Geometry: final body of the model. Coordinates: model frame, mm. A direction names the side the tool comes from. Coordinates: 2 decimals unless noted, no trailing zeros. Order: outer loops, then holes, each group sorted by start corner. A loop starts at its lowest first (then second) coordinate and runs counter-clockwise, first axis right, second up. Notation, with made-up numbers: M 21.25,30.25 L 33.25,30.25 A23 ccw 33.25,38.25 Z; hole C 15.25,58.5 d3. An arc over 180 degrees is marked long. Write item = value, one per line.
from build123d import *

# Parameters (mm, degrees)
SKETCH_1_R          = 10.15
SKETCH_1_R_2        = 1.5
EXTRUDE_1_DEPTH     = 15
SKETCH_2_W          = 12
SKETCH_2_H          = 38
CUT_EXTRUDE_1_DEPTH = 30
CHAMFER_1_SIZE      = 1.5
CUT_EXTRUDE_2_REACH = 56.047
SKETCH_3_R          = 1.6


with BuildPart() as part:
    # ｽｹｯﾁ1 → ﾎﾞｽ - 押し出し1 (new body)
    with BuildSketch(Plane.XY):
        with BuildLine():
            Line((-18.126155741, -8.452365235), (-31.860019201, 21))
            Line((-31.860019201, 21), (31.860019201, 21))
            Line((31.860019201, 21), (18.126155741, -8.452365235))
            ThreePointArc((18.126155741, -8.452365235), (0, -20), (-18.126155741, -8.452365235))
        make_face()
        Circle(SKETCH_1_R, mode=Mode.SUBTRACT)
        with Locations((-9.192388155, 9.192388155)):
            Circle(SKETCH_1_R_2, mode=Mode.SUBTRACT)
        with Locations((9.192388155, 9.192388155)):
            Circle(SKETCH_1_R_2, mode=Mode.SUBTRACT)
        with Locations((-9.192388155, -9.192388155)):
            Circle(SKETCH_1_R_2, mode=Mode.SUBTRACT)
        with Locations((9.192388155, -9.192388155)):
            Circle(SKETCH_1_R_2, mode=Mode.SUBTRACT)
    extrude(amount=EXTRUDE_1_DEPTH)

    # ｽｹｯﾁ2 → ｶｯﾄ - 押し出し1 (cut, symmetric)
    with BuildSketch(Plane(origin=(0, 0, 0), x_dir=(0, 0, -1), z_dir=(1, 0, 0))):
        with Locations((-6, -1)):
            Rectangle(SKETCH_2_W, SKETCH_2_H)
    extrude(amount=CUT_EXTRUDE_1_DEPTH, both=True, mode=Mode.SUBTRACT)

    # 面取り1
    chamfer_1_edges = [part.edges().sort_by_distance(p)[0] for p in [
        (0, 18, 12),
    ]]
    chamfer(chamfer_1_edges, length=CHAMFER_1_SIZE)

    # ｽｹｯﾁ3 → ｶｯﾄ - 押し出し2 (cut, up to next)
    with BuildSketch(Plane(origin=(0, 21, 0), x_dir=(1, 0, 0), z_dir=(0, 1, 0)), mode=Mode.PRIVATE) as cut_extrude_2_sk1:
        with Locations(Location((-20, -7.5, 0), (0, 0, 270))):
            Circle(SKETCH_3_R)
    cut_extrude_2_tool1 = extrude(cut_extrude_2_sk1.sketch, amount=-CUT_EXTRUDE_2_REACH, mode=Mode.PRIVATE) & part.part
    # ｽｹｯﾁ3 → ｶｯﾄ - 押し出し2 (cut, up to next)
    with BuildSketch(Plane(origin=(0, 21, 0), x_dir=(1, 0, 0), z_dir=(0, 1, 0)), mode=Mode.PRIVATE) as cut_extrude_2_sk2:
        with Locations(Location((20, -7.5, 0), (0, 0, 270))):
            Circle(SKETCH_3_R)
    cut_extrude_2_tool2 = extrude(cut_extrude_2_sk2.sketch, amount=-CUT_EXTRUDE_2_REACH, mode=Mode.PRIVATE) & part.part
    add(cut_extrude_2_tool1.solids().sort_by_distance((-20, 21, 7.5))[0], mode=Mode.SUBTRACT)
    add(cut_extrude_2_tool2.solids().sort_by_distance((20, 21, 7.5))[0], mode=Mode.SUBTRACT)


solid = part.part
1) Mould query, pull axis Z, two halves, no side actions, for faces 1 (the face through (8.867, -10.657, 13.479)), 2 (the face through (0.4, 17.2, 11.3)), 3 (the face through (21.586, 19.521, 7.292)). Classes: pulls with the +Z half, pulls with the -Z half, needs draft (parallel to the pull), parting line crosses it, or undercut.
Numbers:
face_1 = needs draft
face_2 = pulls with the -Z half
face_3 = undercut
2) Section D-D, the plane x = -9. Return loops of the section in (y, z), and give its area (3 significant figures).
Numbers:
outline = M -17.86,12 L -10.68,12 L -10.68,15 L -17.86,15 Z; M -7.7,12 L -4.69,12 L -4.69,15 L -7.7,15 Z; M 4.69,12 L 7.7,12 L 7.7,15 L 4.69,15 Z; M 10.68,12 L 16.5,12 L 18,10.5 L 18,0 L 21,0 L 21,15 L 10.68,15 Z
area = 108 mm²
3) Section A-A, the plane z = 7.5. Return loops of the section in (x, y).
Numbers:
outline = M -31.86,21 L -30,17.01 L -30,18 L -21.6,18 L -21.6,21 Z; M -18.4,18 L 18.4,18 L 18.4,21 L -18.4,21 Z; M 21.6,18 L 30,18 L 30,17.01 L 31.86,21 L 21.6,21 Z
4) Line query: L1, parallel to X at y = 19.45, z = 7.5; L2, parallel to Y at x = 20, z = 4.5; L3, parallel to Y at x = 0, z = 14. Output: solid intervals per line, ascending.
Numbers:
L1 = -31.14 to -21.6, -18.4 to 18.4, 21.6 to 31.14
L2 = 18 to 21
L3 = -20 to -10.15, 10.15 to 21
5) Section B-B, the plane x = 0. Return loops of the section in (y, z), and give its area (3 significant figures).
Numbers:
outline = M -20,12 L -10.15,12 L -10.15,15 L -20,15 Z; M 10.15,12 L 16.5,12 L 18,10.5 L 18,0 L 21,0 L 21,15 L 10.15,15 Z
area = 99.2 mm²
6) Set-up query: faces 4 (the face through (7.5, 9.9, 15)), 5 (the face through (0, 18, 5)), 6 (the face through (-6, 10, 12)). Return all of +Z, -Z, +X, -X, +Y, -Y with unobstructed straight access to the full face (end or side cutting, diameter ignored); none if empty.
Numbers:
face_4 = +Z, +X, -X, +Y, -Y
face_5 = -Z, -Y
face_6 = -Z, +X, -X, -Y
7) Section C-C, the plane y = -7. Return loops of the section in (x, z), and give its area (3 significant figures).
Numbers:
outline = M -18.8,12 L -7.35,12 L -7.35,15 L -18.8,15 Z; M 7.35,12 L 18.8,12 L 18.8,15 L 7.35,15 Z
area = 68.7 mm²
8) Pin query (flat end, axial travel): pin 1 (8 mm diameter, centred on x = 23, y = -9, fed in from +Z); pin 2 (5 mm diameter, centred on x = 7, z = 5, fed in from -Y); pin 3 (1.1 mm diameter, centred on y = 17.5, z = 6.5, fed in from +X); pin 4 (12 mm diameter, centred on x = -18, y = -10, fed in from -Z). Return the tip coordinate at first contact, or that it passes through.
Numbers:
pin_1 = through
pin_2 = 18
pin_3 = 30.48
pin_4 = 12
